Build history of the part. All positions in model axes, mm. A direction names the side the tool comes from. Round coordinates to 2 decimals unless told otherwise and drop trailing zeros. Write each loop counter-clockwise with the first axis right and the second up, starting at its lowest first coordinate (ties: lowest second). Pieces come first, ordered by that corner, then holes. Notation, with made-up numbers: (82.5, 85.25) - (121.5, 85.25) arc R26 ccw to (121.5, 121.25) - close; hole circle Ø6 at (17.5, -4). An arc over 180 degrees is marked (long way). One line per question, with ' | ' between items.
from build123d import *

# Parameters (mm, degrees)
BOSS_EXTRUDE1_DEPTH              = 19.05
TAPPED_HOLE_FOR_8_32_HELICOIL1_D = 4.3942
F_1_4_20_TAPPED_HOLE1_D          = 5.1054
F_1_4_CLEARANCE_HOLE1_D          = 7.14248
F_1_4_CLEARANCE_HOLE1_DEPTH      = 12.7
F_1_4_CLEARANCE_HOLE1_TIP        = 2.145817477
CHAMFER2_SIZE                    = 3
CHAMFER3_SIZE                    = 50
FILLET2_R                        = 2


with BuildPart() as part:
    # Sketch1 → Boss-Extrude1 (new body)
    with BuildSketch(Plane.XY):
        with BuildLine():
            Line((78, 0), (78, -17.4))
            Line((78, -17.4), (137, -17.4))
            Line((137, -17.4), (137, -11.05))
            Line((137, -11.05), (120, -11.05))
            Line((120, -11.05), (120, 93))
            Line((120, 93), (0, 93))
            Line((0, 93), (0, 78))
            ThreePointArc((0, 78), (55.154328933, 55.154328933), (78, 0))
        make_face()
    extrude(amount=BOSS_EXTRUDE1_DEPTH)

    # Tapped Hole for #8-32 Helicoil1 (through all)
    with Locations(Plane.XY.offset(19.05)):
        with Locations((21.352571221, 79.688880669), (58.336309448, 58.336309448), (79.688880669, 21.352571221)):
            Hole(TAPPED_HOLE_FOR_8_32_HELICOIL1_D / 2)

    # 1/4-20 Tapped Hole1 (through all)
    with Locations(Plane.XY.offset(19.05)):
        with Locations((108, 20.7), (108, -4.7)):
            Hole(F_1_4_20_TAPPED_HOLE1_D / 2)

    # 1/4 Clearance Hole1
    with Locations(Plane(origin=(0, -11.05, 0), x_dir=(1, 0, 0), z_dir=(0, 1, 0))):
        with Locations((130.5, -9.525)):
            Hole(F_1_4_CLEARANCE_HOLE1_D / 2, depth=F_1_4_CLEARANCE_HOLE1_DEPTH)
            with Locations((0, 0, -(F_1_4_CLEARANCE_HOLE1_DEPTH + F_1_4_CLEARANCE_HOLE1_TIP / 2))):  # 118° drill point
                Cone(0, F_1_4_CLEARANCE_HOLE1_D / 2, F_1_4_CLEARANCE_HOLE1_TIP, mode=Mode.SUBTRACT)

    # Chamfer2
    chamfer2_edges = [part.edges().sort_by_distance(p)[0] for p in [
        (78, -17.4, 9.525),
    ]]
    chamfer(chamfer2_edges, length=CHAMFER2_SIZE)

    # Chamfer3
    chamfer3_edges = [part.edges().sort_by_distance(p)[0] for p in [
        (120, 93, 9.525),
    ]]
    chamfer(chamfer3_edges, length=CHAMFER3_SIZE)

    # Fillet2
    fillet2_edges = [part.edges().sort_by_distance(p)[0] for p in [
        (120, -11.05, 9.525),
        (70, 93, 9.525),
        (120, 43, 9.525),
    ]]
    fillet(fillet2_edges, radius=FILLET2_R)

    # Mirror2: part across plane


with BuildPart() as part_1:
    add(part.part)
    add(part.part.mirror(Plane(origin=(0, 0, 0), x_dir=(0, 0, 1), z_dir=(1, 0, 0))))


solid = part_1.part
Q1. Drop flat-ended pins along their axis: pin 1 (1 mm diameter, centred on y = 56.5, z = 11, fed in from +X); pin 2 (7 mm diameter, centred on x = 21.35, y = 79.69, fed in from -Z); pin 3 (7.5 mm diameter, centred on x = -129.5, z = 5, fed in from +Y); pin 4 (3 mm diameter, centred on x = 108, y = 20.7, fed in from +Z). Give the stop position or say it passes through.
Found:
pin 1: x = 107 | pin 2: z = 0 | pin 3: y = -11.05 | pin 4: through
Q2. Saw through at D-D, the plane z = 16.25. State how many separate pieces and enclosed holes the cut face has, then the cut area to 3 significant figures.
Found:
separate pieces: 1 | enclosed holes: 10 | area: 11,800 mm^2
Q3. Which spindle directions (+Z, -Z, +X, -X, +Y, -Y) get a long thin tool onto all of the face, cutting with end or side? Do faces 5 (the flat face through (120, 16, 9)), 6 (the flat face through (-120, 16, 9)), 7 (the flat face through (-78, -7, 9)). Say none if no direction does.
Found:
face 5: +Z, -Z, +X, +Y | face 6: +Z, -Z, -X, +Y | face 7: +Z, -Z, -Y
Q4. Saw through at B-B, the plane x = -130.5. List the corners of the cut face in (y, z).
Found:
outline: (-17.4, 0) - (-11.05, 0) - (-11.05, 5.95) - (-17.4, 5.95) - close; (-17.4, 13.1) - (-11.05, 13.1) - (-11.05, 19.05) - (-17.4, 19.05) - close
Q5. Pull direction X, two halves, no side cores. Call faces 1 (the flat face through (78, -7, 9)), 2 (the flat face through (126, -11.05, 9)), 3 (the flat face through (-95, 68, 9)), 4 (the cylindrical face through (110.55, -4.59, 9.39)): +X half, -X half, draft (parallel to the pull), parting line (faces both ways), or undercut.
Found:
face 1: undercut | face 2: draft | face 3: -X half | face 4: undercut
Q6. Drill centre lines: L1, parallel to X at y = 0, z = 3.5; L2, parallel to Y at x = 108, z = 11.25; L3, parallel to X at y = 9, z = 15.75. Where is each one in solid material? Low to high. Write a range as from..to.
Found:
L1: -120..-78, 78..120 | L2: -17.4..-7.25, -2.15..18.15, 23.25..55 | L3: -120..-77.48, 77.48..120
Q7. Saw through at C-C, the plane x = 108. List the corners of the cut face in (y, z).
Found:
outline: (-17.4, 0) - (-7.25, 0) - (-7.25, 19.05) - (-17.4, 19.05) - close; (-2.15, 0) - (18.15, 0) - (18.15, 19.05) - (-2.15, 19.05) - close; (23.25, 0) - (55, 0) - (55, 19.05) - (23.25, 19.05) - close
Q8. Saw through at A-A, the plane y = -4.7. List the corners of the cut face in (x, z), then the cut area to 3 significant figures.
Found:
outline: (-120, 0) - (-110.55, 0) - (-110.55, 19.05) - (-120, 19.05) - close; (-105.45, 0) - (-78, 0) - (-78, 19.05) - (-105.45, 19.05) - close; (78, 0) - (105.45, 0) - (105.45, 19.05) - (78, 19.05) - close; (110.55, 0) - (120, 0) - (120, 19.05) - (110.55, 19.05) - close | area: 1,410 mm^2
